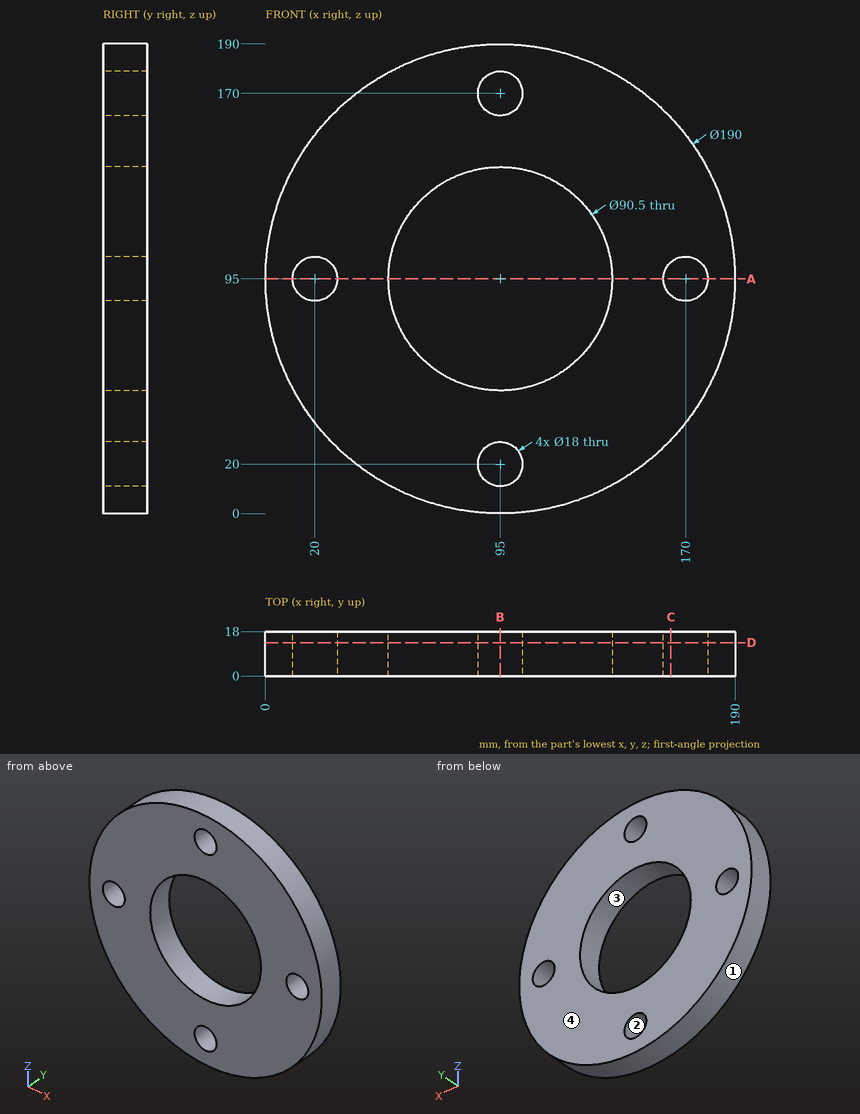
Verification items for this drawing (mm, ordinates from the low corner). Coordinates: 2 decimals unless noted, no trailing zeros. Order: outer loops, then holes, each group sorted by start corner. A loop starts at its lowest first (then second) coordinate and runs counter-clockwise, first axis right, second up. Notation, with made-up numbers: M -16,-10.75 L 20,-10.75 A16 ccw 20,6.25 Z; hole C 13.25,29.5 d10. An arc over 180 degrees is marked long. Write each question's results on one line, items separated by ' | '.
1) Section check D-D on y = 13.5. Record the cut outline in (x, z).
Solved:
outline: C 95,95 d190; hole C 20,95 d18; hole C 95,95 d90.5; hole C 95,20 d18; hole C 95,170 d18; hole C 170,95 d18
2) Section check C-C on x = 164. Record the cut outline in (y, z).
Solved:
outline: M 0,29.7 L 18,29.7 L 18,88.29 L 0,88.29 Z; M 0,101.71 L 18,101.71 L 18,160.3 L 0,160.3 Z
3) Gauge pin test, flat ends, axial feed: pin 1 Ø14.5 at (x, z) = (20, 95) entering from +Y; pin 2 Ø1.5 at (x, y) = (99.5, 8.5) entering from -Z; pin 3 Ø1 at (y, z) = (8, 112) entering from +X; pin 4 Ø4 at (x, y) = (144.5, 4) entering from +Z. Record the tip position at first contact, or that the pin passes through.
Solved:
pin 1: passes through | pin 2: stops at z = 0.07 | pin 3: stops at x = 188.56 | pin 4: stops at z = 177.27
4) Release check for a two-part mould opening along X. For the marked faces 1, 2, 3 and 4 record: pulls with the +X half, pulls with the -X half, needs draft (parallel to the pull), parting line crosses it, or undercut.
Solved:
face 1: parting line crosses it | face 2: undercut | face 3: undercut | face 4: needs draft
5) Scan lines: line 1 along Z through (x, y) = (95, 12.25); line 2 along X through (y, z) = (3.75, 103); line 3 along X through (y, z) = (1, 101.5). Record each from-to range of solid material in increasing order. Write a range as [from, to].
Solved:
line 1: z = [0, 11], [29, 49.75], [140.25, 161], [179, 190] | line 2: x = [0.34, 15.88], [24.12, 50.46], [139.54, 165.88], [174.12, 189.66] | line 3: x = [0.22, 13.78], [26.22, 50.22], [139.78, 163.78], [176.22, 189.78]
6) Section check A-A on z = 95. Record the cut outline in (x, y), plus the area to 3 significant figures.
Solved:
outline: M 0,0 L 11,0 L 11,18 L 0,18 Z; M 29,0 L 49.75,0 L 49.75,18 L 29,18 Z; M 140.25,0 L 161,0 L 161,18 L 140.25,18 Z; M 179,0 L 190,0 L 190,18 L 179,18 Z | area: 1,140 mm²
7) Section check B-B on x = 95. Record the cut outline in (y, z).
Solved:
outline: M 0,0 L 18,0 L 18,11 L 0,11 Z; M 0,29 L 18,29 L 18,49.75 L 0,49.75 Z; M 0,140.25 L 18,140.25 L 18,161 L 0,161 Z; M 0,179 L 18,179 L 18,190 L 0,190 Z
